Can you work these out from the model? Positions are in its coordinate system, mm. A direction names the side the tool comes from. Round coordinates to 2 decimals unless told otherwise and drop trailing zeros. Order: outer loops, then holes, each group sorted by start corner. A loop starts at its lowest first (then second) coordinate and runs counter-clockwise, first axis right, second up.
Q1. We'd pull the mould along X, two halves only. Please class faces 1 (the face through (41.5, 0, 6)), 2 (the face through (32, -3, 6)), 3 (the face through (-41.5, 0, 6)), 4 (the face through (-1, -7, 0)): pulls with the +X half, pulls with the -X half, needs draft (parallel to the pull), parting line crosses it, or undercut.
Q2. If we section it at D-D (y = 12): Please give me the cut outline in (x, z).
Q3. If we section it at B-B (x = 35): Please give me the cut outline in (y, z), plus the area to 3 significant figures.
Q4. If we section it at C-C (y = -0.5): Please give me the cut outline in (x, z).
Q5. Will this pin go through, and if not, where does the flat tip stop? P1, Ø4, axis at x = -32.5, z = 7.5, coming from the +Y side.
Q6. For faces 5 (the face through (-1, 16.5, 6)), 6 (the face through (-32.7, 10.5, 8.3)), which set-ups out of +Z, -Z, +X, -X, +Y, -Y let a thin tool reach every point of the face, with its end or its side?
Q7. If I drill on line 1 (X direction, y = 8, z = 6); line 2 (X direction, y = 13.9, z = 6); line 3 (X direction, y = -1.5, z = 6), over which ranges is the centre line in solid material (lowest first)?
Q8. If we section it at A-A (z = 6): Please give me the cut outline in (x, y), plus the area to 3 significant figures.
from build123d import *

# Parameters (mm, degrees)
SKETCH1_W           = 83
SKETCH1_H           = 33
BOSS_EXTRUDE1_DEPTH = 12
SKETCH2_R           = 5
SKETCH2_R_2         = 6
CUT_EXTRUDE1_DEPTH  = 13
SKETCH3_R           = 3
CUT_EXTRUDE2_DEPTH  = 34
SKETCH4_R           = 5.25
CUT_EXTRUDE3_DEPTH  = 6


with BuildPart() as part:
    # Sketch1 → Boss-Extrude1 (new body)
    with BuildSketch(Plane.XY):
        Rectangle(SKETCH1_W, SKETCH1_H)
    extrude(amount=BOSS_EXTRUDE1_DEPTH)

    # Sketch2 → Cut-Extrude1 (cut, through all)
    with BuildSketch(Plane.XY.offset(12)):
        with Locations((0, 1.5)):
            Circle(SKETCH2_R)
        with Locations((-23, 1.5)):
            Circle(SKETCH2_R_2)
        with Locations((23, 1.5)):
            Circle(SKETCH2_R_2)
    extrude(amount=-CUT_EXTRUDE1_DEPTH, mode=Mode.SUBTRACT)

    # Sketch3 → Cut-Extrude2 (cut, through all)
    with BuildSketch(Plane(origin=(0, 16.5, 0), x_dir=(1, 0, 0), z_dir=(0, 1, 0))):
        with Locations((-35, -6)):
            Circle(SKETCH3_R)
        with Locations((35, -6)):
            Circle(SKETCH3_R)
    extrude(amount=-CUT_EXTRUDE2_DEPTH, mode=Mode.SUBTRACT)

    # Sketch4 → Cut-Extrude3 (cut)
    with BuildSketch(Plane(origin=(0, 16.5, 0), x_dir=(1, 0, 0), z_dir=(0, 1, 0))):
        with Locations((-35, -6)):
            Circle(SKETCH4_R)
        with Locations((35, -6)):
            Circle(SKETCH4_R)
    extrude(amount=-CUT_EXTRUDE3_DEPTH, mode=Mode.SUBTRACT)


solid = part.part
Solution:
1. face 1: pulls with the +X half
1. face 2: undercut
1. face 3: pulls with the -X half
1. face 4: needs draft
2. outline: (-41.5, 0) - (41.5, 0) - (41.5, 12) - (-41.5, 12) - close; hole circle Ø10.5 at (-35, 6); hole circle Ø10.5 at (35, 6)
3. outline: (-16.5, 0) - (16.5, 0) - (16.5, 0.75) - (10.5, 0.75) - (10.5, 3) - (-16.5, 3) - close; (-16.5, 9) - (10.5, 9) - (10.5, 11.25) - (16.5, 11.25) - (16.5, 12) - (-16.5, 12) - close
3. area: 171 mm2
4. outline: (-41.5, 0) - (-28.66, 0) - (-28.66, 12) - (-41.5, 12) - close; (-17.34, 0) - (-4.58, 0) - (-4.58, 12) - (-17.34, 12) - close; (4.58, 0) - (17.34, 0) - (17.34, 12) - (4.58, 12) - close; (28.66, 0) - (41.5, 0) - (41.5, 12) - (28.66, 12) - close; hole circle Ø6 at (-35, 6); hole circle Ø6 at (35, 6)
5. P1: stops at y = 10.5
6. face 5: +Z, -Z, +X, -X, +Y
6. face 6: +Y
7. line 1: x = -41.5 to -38, -32 to 32, 38 to 41.5
7. line 2: x = -41.5 to -40.25, -29.75 to 29.75, 40.25 to 41.5
7. line 3: x = -41.5 to -38, -32 to -28.2, -17.8 to -4, 4 to 17.8, 28.2 to 32, 38 to 41.5
8. outline: (-41.5, -16.5) - (-38, -16.5) - (-38, 10.5) - (-40.25, 10.5) - (-40.25, 16.5) - (-41.5, 16.5) - close; (-32, -16.5) - (32, -16.5) - (32, 10.5) - (29.75, 10.5) - (29.75, 16.5) - (-29.75, 16.5) - (-29.75, 10.5) - (-32, 10.5) - close; (38, -16.5) - (41.5, -16.5) - (41.5, 16.5) - (40.25, 16.5) - (40.25, 10.5) - (38, 10.5) - close; hole circle Ø12 at (-23, 1.5); hole circle Ø10 at (0, 1.5); hole circle Ø12 at (23, 1.5)
8. area: 1,980 mm2
